The model under review builds one solid part; all positions refer to its coordinate system, in mm. Face numbers are marked on the shaded views. Round coordinates to 2 decimals unless told otherwise and drop trailing zeros. Write each loop counter-clockwise with the first axis right and the second up, starting at its lowest first coordinate (ties: lowest second). Pieces come first, ordered by that corner, then holes.
Item 1: To check wall thickness, follow L1, parallel to Z at x = 0, y = 3.5. State the ranges of the line that lie inside material, in increasing order.
Item 2: Draft analysis for pull direction Y (two halves, no side actions). For the marked faces 1, 2 and 3, state which applies: +Y half, -Y half, draft (parallel to the pull), parting line (faces both ways), or undercut.
Item 3: Clearance check with flat-ended pins moving along their axes: pin 1 Ø1 at (x, y) = (69.5, -34) entering from -Z; pin 2 Ø1.5 at (y, z) = (-39.5, -1.5) entering from -X; pin 3 Ø1.5 at (x, z) = (66.5, -2) entering from +Y. State where each tip first meets the part, or that it passes through.
Item 4: Add section A-A (y = 3). Give the boundary of the cut face in (x, z).
Item 5: Add section B-B (x = 49). Give the boundary of the cut face in (y, z), plus the area to 3 significant figures.
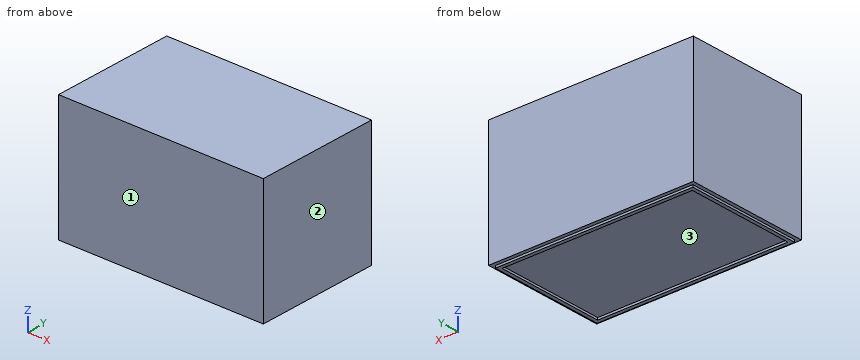
```python
from build123d import *

# Parameters (mm, degrees)
F0_W     = 280
F0_H     = 170
F1_DEPTH = 170
F2_W     = 270
F2_H     = 160
F2_W_2   = 260
F2_H_2   = 150
F3_DEPTH = 3


with BuildPart() as f1:
    # F0 (on Top) → F1 (new body)
    with BuildSketch(Plane.XY):
        Rectangle(F0_W, F0_H)
    extrude(amount=F1_DEPTH)

    # F2 (on face) → F3 (join)
    with BuildSketch(Plane(origin=(0, 0, 0), x_dir=(1, 0, 0), z_dir=(0, 0, -1))):
        Rectangle(F2_W, F2_H)
        Rectangle(F2_W_2, F2_H_2, mode=Mode.SUBTRACT)
    extrude(amount=F3_DEPTH)


solid = f1.part
```
Numbers:
1. L1: z = 0 to 170
2. face 1: -Y half
2. face 2: draft
2. face 3: undercut
3. pin 1: stops at z = 0
3. pin 2: stops at x = -135
3. pin 3: stops at y = 80
4. outline: (-140, 0) - (-135, 0) - (-135, -3) - (-130, -3) - (-130, 0) - (130, 0) - (130, -3) - (135, -3) - (135, 0) - (140, 0) - (140, 170) - (-140, 170) - close
5. outline: (-85, 0) - (-80, 0) - (-80, -3) - (-75, -3) - (-75, 0) - (75, 0) - (75, -3) - (80, -3) - (80, 0) - (85, 0) - (85, 170) - (-85, 170) - close
5. area: 28,900 mm2
